Read the model definition and answer for the solid it produces. Units are mm, in the model's axes. Coordinates: 2 decimals unless noted, no trailing zeros. Order: outer loops, then holes, each group sorted by start corner. A loop starts at its lowest first (then second) coordinate and runs counter-clockwise, first axis right, second up. Notation, with made-up numbers: M 22,-8.5 L 31,-8.5 A32 ccw 31,27.5 Z; hole C 3.25,32 d10. An arc over 180 degrees is marked long. Use a Markdown table: item, result. Add a question column.
1) Find section D-D on x = 9.5. Write down the section's boundary in (y, z), plus the area to 3 significant figures.
2) Find section A-A on x = -2.5. Write down the section's boundary in (y, z) (3 decimals).
3) Find section B-B on y = 3.5. Write down the section's boundary in (x, z) (3 decimals).
4) Find section C-C on x = 12.6. Write down the section's boundary in (y, z) (3 decimals), plus the area to 3 significant figures.
5) Find the intervals of material crossed by probe 1 along Z at (x, y) = (-2.5, 3.65) (3 decimals); probe 2 along X at (y, z) = (3.3, 7.5); probe 3 along Z at (x, y) = (13.5, 4.45), in increasing order. Write a range as [from, to].
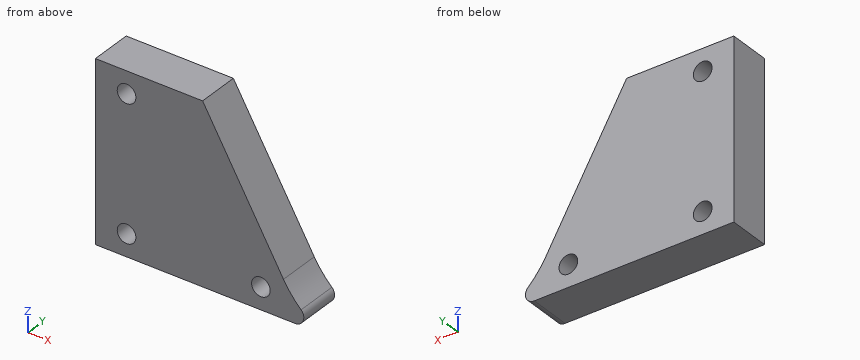
Autodesk Inventor part; units mm, degrees
ref_plane "YZ Plane" through (0, 0, 0) normal (1, 0, 0) x (0, 1, 0)
ref_plane "XZ Plane" through (0, 0, 0) normal (0, 1, 0) x (-1, 0, 0)
ref_plane "XY Plane" through (0, 0, 0) normal (0, 0, 1) x (1, 0, 0)
sketch "Sketch1" plane through (0, 0, 0) normal (0, 1, 0) x (-1, 0, 0)
  line L0 (4, 10) -> (-19.4211, 10)
  line L1 (-19.4211, -10) -> (4, -10)
  line L2 (4, -10) -> (4, 10)
  arc A0 (-19.4211, -10) -> (-19.4211, 10) centre (-25.1, 0) ccw
  line L3 (4, -10) -> (6, -10)
  line L4 (6, -10) -> (6, 10)
  line L5 (6, 10) -> (4, 10)
  line L6 (4, 10) -> (4, -10)
  point P0 (0, 0)
  dimension "d0" = 20
  dimension "d2" = 4
  dimension "d3" = 10
  dimension "d6" = 10
  dimension "d7" = 23
  dimension "d8" = 29.1
  dimension "d11" = 23.4211
  dimension "d12" = 20
  dimension "d13" = 2
extrude "Extrusion1" add sketch "Sketch1" along normal blind 4.71
fillet "Fillet1" radius 1 2 edges at (19.4211, 2.355, -10) (19.4211, 2.355, 10)
sketch "Sketch3" plane through (0, 0, 0) normal (0, -1, 0) x (1, 0, 0)
  circle A0 centre (-2.5, -7.525) radius 1.05
  circle A1 centre (12.6, -7.525) radius 1.05
  circle A2 centre (12.6, 7.525) radius 1.05
  circle A3 centre (-2.5, 7.525) radius 1.05
  point P0 (0, 0)
hole "Hole2" at (-2.5, 0, -7.525) at (-2.5, 0, 7.525) at (12.6, 0, 7.525) at (12.6, 0, -7.525) direction (0, 1, 0) diameter 2.1 end through all
sketch "Sketch4" plane through (0, 0, 0) normal (0, -1, 0) x (1, 0, 0)
  line L0 (1.4953, 17.8846) -> (19.0725, -12.5601)
  arc A0 (17.1193, 8.28) -> (17.1193, -8.28) centre (25.1, 0) ccw
  arc A1 (17.1193, 8.28) -> (16.4253, 10) centre (16.4253, 9) ccw
  line L1 (-6, 10) -> (16.4253, 10)
  point P0 (0, 0)
  point P1 (6.0474, 10)
  point P2 (15.1407, -5.75)
  dimension "d29" = 60
extrude "Extrusion2" cut sketch "Sketch4" against normal up to next
properties part number "3D_printed_part"
Check result:
| question | item | result |
|---|---|---|
| 1 | outline | M 0,-10 L 4.71,-10 L 4.71,4.02 L 0,4.02 Z |
| 1 | area | 66.0 mm2 |
| 2 | outline | M 0,-10 L 4.71,-10 L 4.71,-8.575 L 0,-8.575 Z; M 0,-6.475 L 4.71,-6.475 L 4.71,6.475 L 0,6.475 Z; M 0,8.575 L 4.71,8.575 L 4.71,10 L 0,10 Z |
| 3 | outline | M -6,-10 L 16.425,-10 A1 ccw 17.119,-8.28 A11.5 cw 15.141,-5.75 L 6.047,10 L -6,10 Z; hole C -2.5,-7.525 d2.1; hole C -2.5,7.525 d2.1; hole C 12.6,-7.525 d2.1 |
| 4 | outline | M 0,-10 L 4.71,-10 L 4.71,-8.575 L 0,-8.575 Z; M 0,-6.475 L 4.71,-6.475 L 4.71,-1.349 L 0,-1.349 Z |
| 4 | area | 30.9 mm2 |
| 5 | probe 1 | z = [-10, -8.575], [-6.475, 6.475], [8.575, 10] |
| 5 | probe 2 | x = [-6, -3.55], [-1.45, 7.49] |
| 5 | probe 3 | z = [-10, -8.07], [-6.98, -2.91] |
